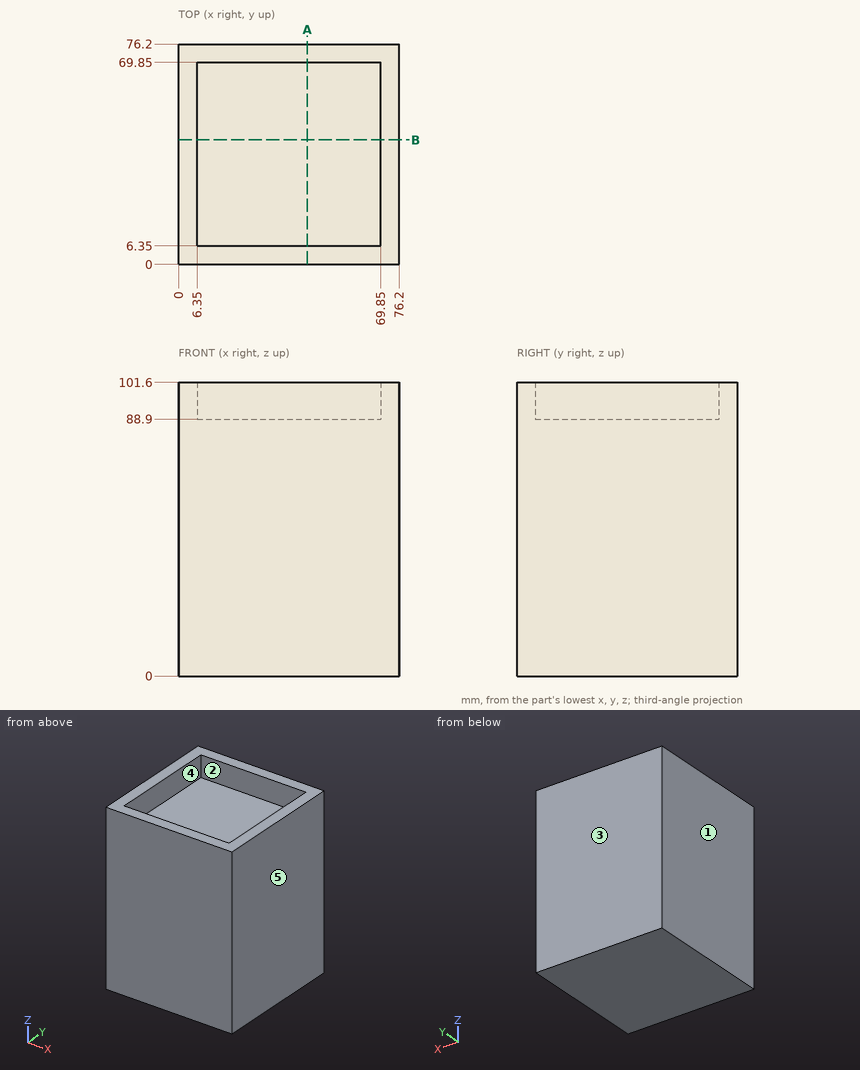
Answer from the drawing. Dimensions are ordinates in mm from the lowest x, y and z of the part. A direction names the side the tool comes from. Give positions to 0.01 mm unless a question says otherwise; leave off trailing zeros. Order: outer loops, then holes, each group sorted by start corner. A loop starts at its lowest first (then second) coordinate and runs counter-clockwise, first axis right, second up.
Item 1: The part is cut by section A-A, the plane x = 44.5. Give the vertices of the cut face in (y, z).
From the geometry:
outline: (0, 0) - (76.2, 0) - (76.2, 101.6) - (69.85, 101.6) - (69.85, 88.9) - (6.35, 88.9) - (6.35, 101.6) - (0, 101.6) - close
Item 2: For a pull along X with two mould halves and no side action, classify the marked faces 3, 4 and 5 as pulls with the +X half, pulls with the -X half, needs draft (parallel to the pull), parting line crosses it, or undercut.
From the geometry:
face 3: needs draft
face 4: undercut
face 5: pulls with the +X half
Item 3: Which of the six approach directions +Z, -Z, +X, -X, +Y, -Y give full straight-line access (tool end or side, diameter ignored) to the marked faces 1 and 2?
From the geometry:
face 1: +Z, -Z, -X, +Y, -Y
face 2: +Z
Item 4: Find the intervals of material crossed by probe 1 along Y at (x, z) = (45.5, 91); probe 2 along Z at (x, y) = (40, 13), in increasing order.
From the geometry:
probe 1: y = 0 to 6.35, 69.85 to 76.2
probe 2: z = 0 to 88.9
Item 5: Given pin 1 Ø4 at (x, y) = (8.5, 13.5) entering from -Z; pin 2 Ø2 at (x, y) = (39, 35.5) entering from +Z, each flat-ended and moving along its own axis, determine where each tip first touches the part or whether it passes through.
From the geometry:
pin 1: stops at z = 0
pin 2: stops at z = 88.9
